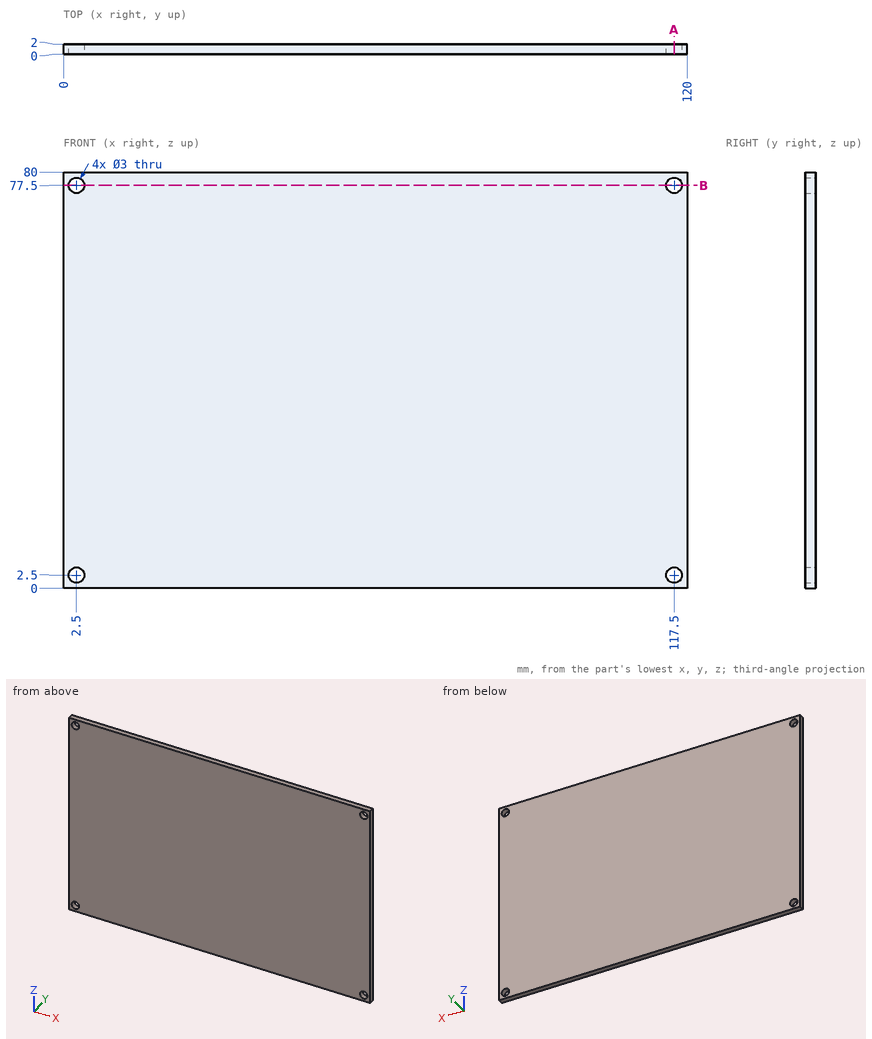
Here's the drawing with two shaded views (mm, measured from the low corner). I have some questions. Give positions to 0.01 mm unless a question says otherwise; leave off trailing zeros. Order: outer loops, then holes, each group sorted by start corner. A loop starts at its lowest first (then second) coordinate and runs counter-clockwise, first axis right, second up. Notation, with made-up numbers: (19, -22.75) - (52, -22.75) arc R14 cw to (52, 2.25) - close; hole circle Ø5 at (73, -29). An arc over 180 degrees is marked (long way). Write each question's results on one line, items separated by ' | '.
1) Please list where these lines run through material, in increasing order: line 1 along X through (y, z) = (1.2, 2.5); line 2 along Z through (x, y) = (117.5, 1.25). Write a range as [from, to].
Final values:
line 1: x = [0, 1], [4, 116], [119, 120] | line 2: z = [0, 1], [4, 76], [79, 80]
2) Suppose I cut it at A-A, the plane x = 117.5. Write out the boundary of the cut face in (y, z).
Final values:
outline: (0, 0) - (2, 0) - (2, 1) - (0, 1) - close; (0, 4) - (2, 4) - (2, 76) - (0, 76) - close; (0, 79) - (2, 79) - (2, 80) - (0, 80) - close
3) I'm going to push a flat-ended pin straight in: pin 1 Ø1.8 at (x, z) = (117.5, 77.5) entering from +Y. Where does the tip first touch, or does it pass through?
Final values:
pin 1: passes through
4) Suppose I cut it at B-B, the plane z = 77.5. Write out the boundary of the cut face in (x, y), then the cut area to 3 significant figures.
Final values:
outline: (0, 0) - (1, 0) - (1, 2) - (0, 2) - close; (4, 0) - (116, 0) - (116, 2) - (4, 2) - close; (119, 0) - (120, 0) - (120, 2) - (119, 2) - close | area: 228 mm^2
